Autodesk Inventor part; units mm, degrees
ref_plane "YZ Plane" through (0, 0, 0) normal (1, 0, 0) x (0, 1, 0)
ref_plane "XZ Plane" through (0, 0, 0) normal (0, 1, 0) x (-1, 0, 0)
ref_plane "XY Plane" through (0, 0, 0) normal (0, 0, 1) x (1, 0, 0)
sketch "Sketch1" plane through (0, 0, 0) normal (0, 0, 1) x (1, 0, 0)
  line L0 (-13.819, 82.4) -> (-7.5425, 82.4)
  line L1 (24.2075, 82.4) -> (30.484, 82.4)
  arc A0 (24.2075, 82.4) -> (-7.5425, 82.4) centre (8.3325, 82.4) ccw
  arc A1 (30.484, 82.4) -> (15.2091, -70) centre (209.6265, -12.5208) ccw
  line L2 (2.5091, -70) -> (15.2091, -70)
  arc A2 (-13.819, 82.4) -> (2.5091, -70) centre (99.9218, 17.5115) ccw
  point P0 (0, 0)
  dimension "d0" = 31.75
  dimension "d1" = 12.7
  dimension "d2" = 152.4
  dimension "d9" = 70
extrude "Extrusion1" add sketch "Sketch1" along normal blind 5.3
sketch "Sketch2" plane through (0, 0, 5.3) normal (0, 0, 1) x (1, 0, 0)
  line L0 (-3.7203, -6.5) -> (27.9202, -6.5)
  line L1 (27.9202, -6.5) -> (27.9202, -11.8)
  line L2 (27.9202, -11.8) -> (-3.7203, -11.8)
  line L3 (-3.7203, -11.8) -> (-3.7203, -6.5)
  line L4 (-7.5425, 82.4) -> (-13.819, 82.4)
  line L5 (-7.5425, 82.4) -> (-13.819, 82.4)
  arc A0 (-13.819, 82.4) -> (2.5091, -70) centre (99.9218, 17.5115) ccw
  line L6 (2.5091, -70) -> (15.2091, -70)
  arc A1 (30.484, 82.4) -> (15.2091, -70) centre (209.6265, -12.5208) ccw
  line L7 (30.484, 82.4) -> (24.2075, 82.4)
  arc A2 (24.2075, 82.4) -> (-7.5425, 82.4) centre (8.3325, 82.4) ccw
  point P0 (0, 0)
  point P1 (6.9797, -6.5)
  dimension "d5" = 5.3
  dimension "d6" = 88.9
  dimension "d10" = 10.7
extrude "Extrusion2" cut sketch "Sketch2" against normal up to surface (5.3 mm away) contours L0 A1 L2 L3 | L0 L1 L2 A1
properties part number "leg"
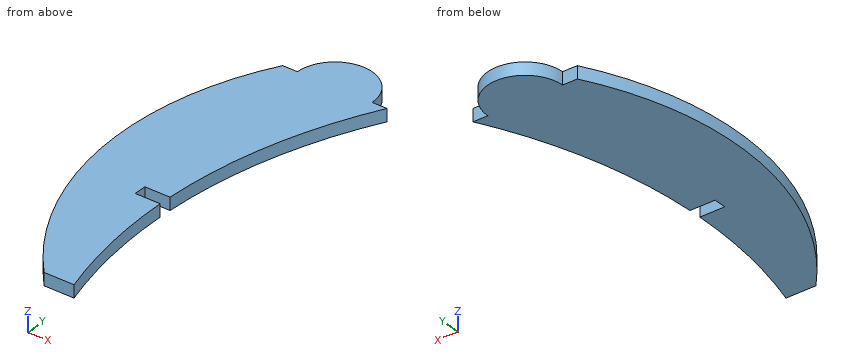
Part model, mm, in its own coordinate system. Give positions to 0.01 mm unless a question says otherwise; leave off trailing zeros. Loops run counter-clockwise (first coordinate to the right, second up) from the corner with the lowest first, then second, coordinate; pieces in that order, holes last.
(1) Band-saw the part on B-B (x = -26). Write the cut outline in (y, z), and give its area (3 significant figures).
Return value:
outline: (-18.42, 0) - (53.44, 0) - (53.44, 5.3) - (-18.42, 5.3) - close
area: 381 mm2
(2) Band-saw the part on C-C (y = 32). Write the cut outline in (x, z), and give its area (3 significant figures).
Return value:
outline: (-30.22, 0) - (11.84, 0) - (11.84, 5.3) - (-30.22, 5.3) - close
area: 223 mm2
(3) Pin check, flat tips, straight feed: pin 1 (1.5 mm diameter, centred on y = -31, z = 1, fed in from -X); pin 2 (2.5 mm diameter, centred on x = 27.5, z = 3.5, fed in from +Y); pin 3 (2.5 mm diameter, centred on x = 0.5, z = 1.5, fed in from +Y). Stop position of each tip, or through.
Return value:
pin 1: stops at x = -22.01
pin 2: stops at y = 82.4
pin 3: stops at y = 96.85
(4) Drill centre lines: line 1 along Y through (x, z) = (6.5, 4.6); line 2 along X through (y, z) = (10, 2.65); line 3 along X through (y, z) = (-49, 2.95). Where is each one in solid material? Low to high.
Return value:
line 1: y = -70 to -11.8, -6.5 to 98.17
line 2: x = -30.81 to 8.14
line 3: x = -12.88 to 10.2
